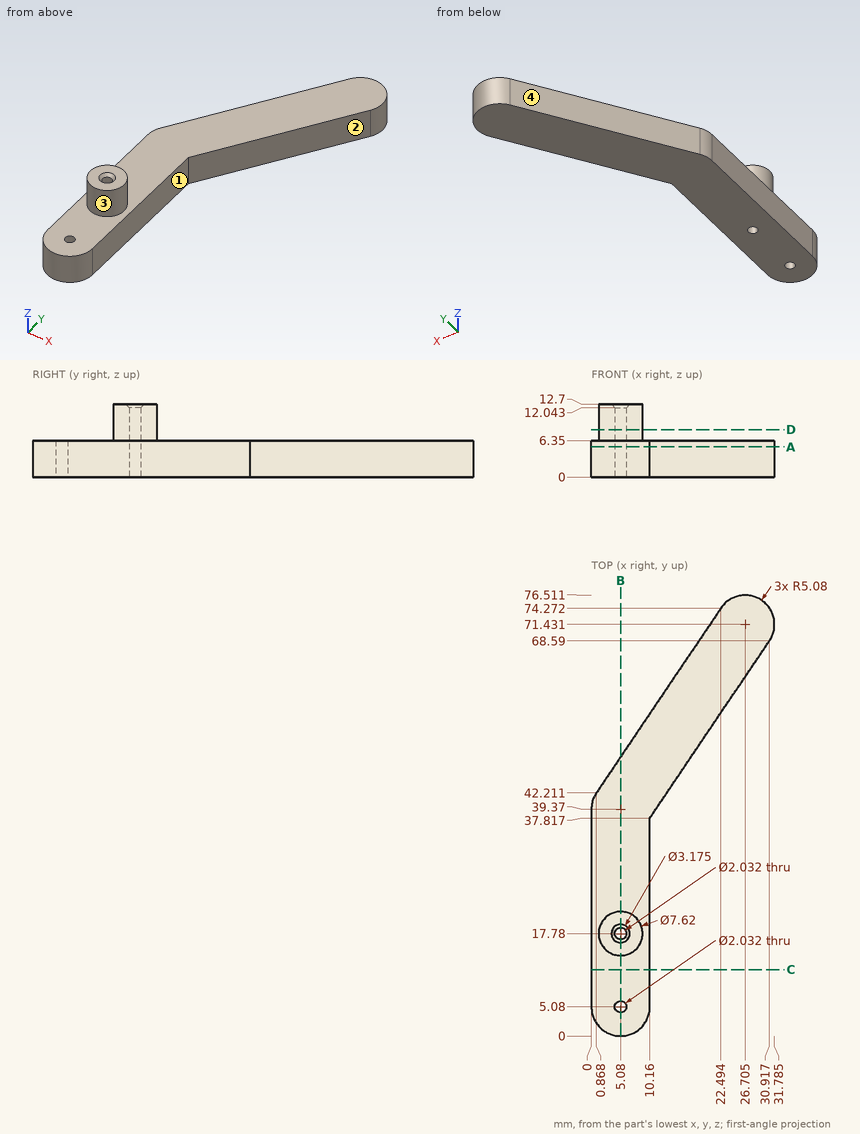
For this review, use the dimensioned drawing (mm, ordinates from the lowest corner) and the shaded views. Coordinates: 2 decimals unless noted, no trailing zeros. Write each loop counter-clockwise with the first axis right and the second up, starting at its lowest first coordinate (ties: lowest second). Pieces come first, ordered by that corner, then holes. Notation, with made-up numbers: (-35, 27.25) - (-22, 27.25) arc R19 cw to (-22, 41.25) - close; hole circle Ø8 at (75, 63). An arc over 180 degrees is marked (long way). Answer as a JSON object with one key per item and string values. Group by question number.
1. Add section A-A (z = 5.25). Give the boundary of the cut face in (x, y) (1 decimal).
2. Mouldability with a two-part tool opening along Y and no side actions: class the marked faces 1, 2, 3 and 4 as pulls with the +Y half, pulls with the -Y half, needs draft (parallel to the pull), parting line crosses it, or undercut.
3. Add section B-B (x = 5.08). Give the number of separate pieces and of enclosed holes in the cut face, plus the area to 3 significant figures.
4. To check wall thickness, follow probe 1 along Y at (x, z) = (5.08, 8.5) (1 decimal); probe 2 along Y at (x, z) = (5.08, 4.5) (1 decimal); probe 3 along X at (y, z) = (33, 2.5). State the ranges of each line that lie inside material, in increasing order.
5. Add section C-C (y = 11.5). Give the boundary of the cut face in (x, z).
6. Clearance check with flat-ended pins moving along their axes: pin 1 Ø2 at (y, z) = (17.5, 8.5) entering from +X; pin 2 Ø2.5 at (x, y) = (5.08, 5.08) entering from +Z; pin 3 Ø3 at (y, z) = (9, 1.5) entering from +X. State where each tip first meets the part, or that it passes through.
7. Add section D-D (z = 8.25). Give the boundary of the cut face in (x, y).
Findings:
{
 "1": {"outline": "(0, 5.1) arc R5.1 ccw to (10.2, 5.1) - (10.2, 37.8) - (30.9, 68.6) arc R5.1 ccw to (22.5, 74.3) - (0.9, 42.2) arc R5.1 ccw to (0, 39.4) - close; hole circle Ø2 at (5.1, 5.1); hole circle Ø2 at (5.1, 17.8)"},
 "2": {"face 1": "needs draft", "face 2": "pulls with the -Y half", "face 3": "parting line crosses it", "face 4": "pulls with the +Y half"},
 "3": {"separate pieces": "3", "enclosed holes": "0", "area": "317 mm²"},
 "4": {"probe 1": "14 to 16.8, 18.8 to 21.6", "probe 2": "0 to 4.1, 6.1 to 16.8, 18.8 to 48.5", "probe 3": "0 to 10.16"},
 "5": {"outline": "(0, 0) - (10.16, 0) - (10.16, 6.35) - (0, 6.35) - close"},
 "6": {"pin 1": "x = 8.89", "pin 2": "z = 6.35", "pin 3": "x = 10.16"},
 "7": {"outline": "circle Ø7.62 at (5.08, 17.78); hole circle Ø2.03 at (5.08, 17.78)"}
}
